For this review, take the finished solid that the model builds, in its own axes (mm). A direction names the side the tool comes from. Give positions to 0.01 mm unless a question says otherwise; leave off trailing zeros. Write each loop counter-clockwise with the first axis right and the second up, starting at its lowest first coordinate (ties: lowest second). Pieces come first, ordered by that corner, then holes.
Q1. We need section D-D (z = -69.5). Write out the cut boundary in (x, y).
Q2. We need section C-C (y = 3.75). Give the number of separate pieces and of enclosed holes in the cut face, then the cut area to 3 significant figures.
Q3. We need section A-A (x = 0). Write out the cut boundary in (y, z).
Q4. We need section B-B (z = -25.5). Write out the cut boundary in (x, y).
Q5. Mouldability with a two-part tool opening along X and no side actions: class faces 1 (the flat face through (-6, 15, -81)), 2 (the flat face through (16.53, 7.4, -79.47)), 3 (the flat face through (-22.155, 7.395, -72.693)) as released by +X, released by -X, zero draft, split by the parting line, or undercut.
Q6. Insertion check: P1, Ø4, axis at y = 7, z = -121, coming from the +X side; P2, Ø5, axis at y = 2.5, z = -120, coming from the -X side; P3, Ø1, axis at x = -18.5, y = 3, coming from the -Z side. Each pin has a flat end and moves straight along its axis. Give the tip position at first contact, or say it passes through.
Q7. Machinability: for faces 4 (the flat face through (-14.993, 7.395, -52.393)), 5 (the conical face through (9.46, 12.62, -129.3)), which of the approach directions +Z, -Z, +X, -X, +Y, -Y give a long, thin tool a straight path to every point of the face, cutting with its end or side? Answer none if there is none.
Q8. For line 1 (X direction, y = 5, z = -150); line 2 (X direction, y = 14.25, z = -52); line 3 (Z direction, x = -12.5, y = 3), list the stretches that pass through material, from the lowest coordinate up.
```python
from build123d import *

# Parameters (mm, degrees)
SKETCH_1_R               = 5
SKETCH_1_R_2             = 15
EXTRUDE_1_DEPTH          = 15
FILLET_1_R               = 3
SKETCH_2_R               = 2.6
CUT_EXTRUDE_1_DEPTH      = 180.107509614
PATTERN_CIRCULAR_5_COUNT = 3
CHAMFER_1_SIZE           = 2.5


with BuildPart() as part:
    # 草图1 → 凸台-拉伸1 (new body)
    with BuildSketch(Plane(origin=(0, 0, 0), x_dir=(1, 0, 0), z_dir=(0, 1, 0))):
        with BuildLine():
            Line((-17.971076762, -1.02), (-26.457418567, 148.498333333))
            ThreePointArc((-26.457418567, 148.498333333), (0, 176.5), (26.457418567, 148.498333333))
            Line((26.457418567, 148.498333333), (17.971076762, -1.02))
            ThreePointArc((17.971076762, -1.02), (0, -18), (-17.971076762, -1.02))
        make_face()
        with Locations(Location((0, 0, 0), (0, 0, 270))):
            Circle(SKETCH_1_R, mode=Mode.SUBTRACT)
        with Locations(Location((0, 150, 0), (0, 0, 270))):
            Circle(SKETCH_1_R_2, mode=Mode.SUBTRACT)
        Polygon((-12.740980954, 12.714849757), (-18.554385191, 115.139490738), (10.712851955, 17.329399023), align=None, mode=Mode.SUBTRACT)
        Polygon((13.283215706, 22.268322657), (18.830257334, 120), (-12, 127), align=None, mode=Mode.SUBTRACT)
    extrude(amount=EXTRUDE_1_DEPTH)

    # 圆角1
    fillet_1_edges = [part.edges().sort_by_distance(p)[0] for p in [
        (-12.740980954, 7.5, -12.714849757),
        (10.712851955, 7.5, -17.329399023),
        (-18.554385191, 7.5, -115.139490738),
        (18.830257334, 7.5, -120),
        (-12, 7.5, -127),
        (13.283215706, 7.5, -22.268322657),
    ]]
    fillet(fillet_1_edges, radius=FILLET_1_R)

    # 草图2 → 切除-拉伸1 (cut, through all)
    with BuildSketch(Plane(origin=(0, 15, 0), x_dir=(1, 0, 0), z_dir=(0, 1, 0))):
        with Locations(Location((-21, 150, 0), (0, 0, 270))):
            Circle(SKETCH_2_R)
        with Locations(Location((21, 150, 0), (0, 0, 270))):
            Circle(SKETCH_2_R)
    cut_extrude_1 = extrude(amount=-CUT_EXTRUDE_1_DEPTH, mode=Mode.SUBTRACT)

    # 阵列(圆周)5: 切除-拉伸1 ×3 about axis
    pattern_circular_5_axis = Axis((0, 0, -150), (0, 1, 0))
    for i in range(1, PATTERN_CIRCULAR_5_COUNT):
        add(cut_extrude_1.rotate(pattern_circular_5_axis, i * 360 / PATTERN_CIRCULAR_5_COUNT), mode=Mode.SUBTRACT)

    # 倒角1
    chamfer_1_edges = [part.edges().sort_by_distance(p)[0] for p in [
        (-12.75166605, 15, -166.886533479),
        (-8.24833395, 15, -130.513466521),
        (-21, 15, -152.6),
        (21, 15, -152.6),
        (8.24833395, 15, -130.513466521),
        (12.75166605, 15, -166.886533479),
    ]]
    chamfer(chamfer_1_edges, length=CHAMFER_1_SIZE)


solid = part.part
```
Computed:
1. outline: (-21.97, 0) - (-15.96, 0) - (-15.96, 15) - (-21.97, 15) - close; (-4.9, 0) - (1.88, 0) - (1.88, 15) - (-4.9, 15) - close; (15.96, 0) - (21.97, 0) - (21.97, 15) - (15.96, 15) - close
2. separate pieces: 1
2. enclosed holes: 10
2. area: 4,770 mm2
3. outline: (0, -176.5) - (15, -176.5) - (15, -165) - (0, -165) - close; (0, -135) - (15, -135) - (15, -124.28) - (0, -124.28) - close; (0, -77.29) - (15, -77.29) - (15, -53.13) - (0, -53.13) - close; (0, -15.22) - (15, -15.22) - (15, -5) - (0, -5) - close; (0, 5) - (15, 5) - (15, 18) - (0, 18) - close
4. outline: (-19.48, 0) - (-13.47, 0) - (-13.47, 15) - (-19.48, 15) - close; (8.27, 0) - (19.48, 0) - (19.48, 15) - (8.27, 15) - close
5. face 1: zero draft
5. face 2: undercut
5. face 3: released by -X
6. P1: stops at x = 25.01
6. P2: stops at x = -24.98
6. P3: stops at z = -169.45
7. face 4: +Y, -Y
7. face 5: +Y
8. line 1: x = -26.5 to -23.6, -18.4 to -15, 15 to 18.4, 23.6 to 26.5
8. line 2: x = -20.98 to -14.97, 0.34 to 6.11, 14.97 to 20.98
8. line 3: z = -173.37 to -169.85, -166.53 to -158.29, -141.71 to -133.47, -130.15 to -92.36, -14.76 to 12.95
